Could you check a few things on this model? Use its own coordinates, in mm. A direction names the side the tool comes from. Give positions to 0.01 mm unless a question says otherwise; leave off trailing zeros. Order: outer loops, then holes, each group sorted by start corner. A loop starts at its lowest first (then second) coordinate and runs counter-clockwise, first axis right, second up. Notation, with made-up numbers: (46, 45.25) -> (75, 45.25) arc R21 cw to (75, 62.25) -> close; hole circle Ø5 at (-27.75, -1.5). An arc over 180 degrees is marked (long way). One line per item, written item: value.
```python
from build123d import *

# Parameters (mm, degrees)
F1_DEPTH = 12.7


with BuildPart() as f1:
    # F0 (on Front) → F1 (new body)
    with BuildSketch(Plane.XZ):
        with BuildLine():
            ThreePointArc((13.700902, 62.328232), (6.890739, 63.44321), (0, 63.816324))
            ThreePointArc((0, 63.816324), (-1.449213, 63.799867), (-2.897679, 63.750503))
            ThreePointArc((-2.897679, 63.750503), (-9.764368, 63.06489), (-16.51688, 61.641836))
            ThreePointArc((-16.51688, 61.641836), (-17.912453, 61.250855), (-19.298787, 60.828283))
            ThreePointArc((-19.298787, 60.828283), (-25.75405, 58.388801), (-31.908162, 55.266558))
            ThreePointArc((-31.908162, 55.266558), (-33.154989, 54.527699), (-34.384715, 53.760716))
            ThreePointArc((-34.384715, 53.760716), (-39.988636, 49.733612), (-45.124956, 45.124956))
            ThreePointArc((-45.124956, 45.124956), (-46.138067, 44.08857), (-47.127381, 43.029445))
            ThreePointArc((-47.127381, 43.029445), (-51.498062, 37.68916), (-55.266558, 31.908162))
            ThreePointArc((-55.266558, 31.908162), (-55.976912, 30.644878), (-56.658395, 29.365788))
            ThreePointArc((-56.658395, 29.365788), (-59.497981, 23.076254), (-61.641836, 16.51688))
            ThreePointArc((-61.641836, 16.51688), (-62.001023, 15.112788), (-62.328232, 13.700902))
            ThreePointArc((-62.328232, 13.700902), (-63.44321, 6.890739), (-63.816324, 0))
            ThreePointArc((-63.816324, 0), (-63.799867, -1.449213), (-63.750503, -2.897679))
            ThreePointArc((-63.750503, -2.897679), (-63.06489, -9.764368), (-61.641836, -16.51688))
            ThreePointArc((-61.641836, -16.51688), (-61.250855, -17.912453), (-60.828283, -19.298787))
            ThreePointArc((-60.828283, -19.298787), (-58.388801, -25.75405), (-55.266558, -31.908162))
            ThreePointArc((-55.266558, -31.908162), (-54.527699, -33.154989), (-53.760716, -34.384715))
            ThreePointArc((-53.760716, -34.384715), (-49.733612, -39.988636), (-45.124956, -45.124956))
            ThreePointArc((-45.124956, -45.124956), (-44.08857, -46.138067), (-43.029445, -47.127381))
            ThreePointArc((-43.029445, -47.127381), (-37.68916, -51.498062), (-31.908162, -55.266558))
            ThreePointArc((-31.908162, -55.266558), (-30.644878, -55.976912), (-29.365788, -56.658395))
            ThreePointArc((-29.365788, -56.658395), (-23.076254, -59.497981), (-16.51688, -61.641836))
            ThreePointArc((-16.51688, -61.641836), (-15.112788, -62.001023), (-13.700902, -62.328232))
            ThreePointArc((-13.700902, -62.328232), (-6.890739, -63.44321), (0, -63.816324))
            ThreePointArc((0, -63.816324), (1.449213, -63.799867), (2.897679, -63.750503))
            ThreePointArc((2.897679, -63.750503), (9.764368, -63.06489), (16.51688, -61.641836))
            ThreePointArc((16.51688, -61.641836), (17.912453, -61.250855), (19.298787, -60.828283))
            ThreePointArc((19.298787, -60.828283), (25.75405, -58.388801), (31.908162, -55.266558))
            ThreePointArc((31.908162, -55.266558), (33.154989, -54.527699), (34.384715, -53.760716))
            ThreePointArc((34.384715, -53.760716), (39.988636, -49.733612), (45.124956, -45.124956))
            ThreePointArc((45.124956, -45.124956), (46.138067, -44.08857), (47.127381, -43.029445))
            ThreePointArc((47.127381, -43.029445), (51.498062, -37.68916), (55.266558, -31.908162))
            ThreePointArc((55.266558, -31.908162), (55.976912, -30.644878), (56.658395, -29.365788))
            ThreePointArc((56.658395, -29.365788), (59.497981, -23.076254), (61.641836, -16.51688))
            ThreePointArc((61.641836, -16.51688), (62.001023, -15.112788), (62.328232, -13.700902))
            ThreePointArc((62.328232, -13.700902), (63.44321, -6.890739), (63.816324, 0))
            ThreePointArc((63.816324, 0), (63.799867, 1.449213), (63.750503, 2.897679))
            ThreePointArc((63.750503, 2.897679), (63.06489, 9.764368), (61.641836, 16.51688))
            ThreePointArc((61.641836, 16.51688), (61.250855, 17.912453), (60.828283, 19.298787))
            ThreePointArc((60.828283, 19.298787), (58.388801, 25.75405), (55.266558, 31.908162))
            ThreePointArc((55.266558, 31.908162), (54.527699, 33.154989), (53.760716, 34.384715))
            ThreePointArc((53.760716, 34.384715), (49.733612, 39.988636), (45.124956, 45.124956))
            ThreePointArc((45.124956, 45.124956), (44.08857, 46.138067), (43.029445, 47.127381))
            ThreePointArc((43.029445, 47.127381), (37.68916, 51.498062), (31.908162, 55.266558))
            ThreePointArc((31.908162, 55.266558), (30.644878, 55.976912), (29.365788, 56.658395))
            ThreePointArc((29.365788, 56.658395), (23.076254, 59.497981), (16.51688, 61.641836))
            ThreePointArc((16.51688, 61.641836), (15.112788, 62.001023), (13.700902, 62.328232))
        make_face()
        with BuildLine():
            ThreePointArc((-45.124956, 45.124956), (-39.988636, 49.733612), (-34.384715, 53.760716))
            Line((-34.384715, 53.760716), (-53.916988, 53.916988))
            Line((-53.916988, 53.916988), (-45.124956, 45.124956))
        make_face()
        with BuildLine():
            ThreePointArc((-31.908162, 55.266558), (-25.75405, 58.388801), (-19.298787, 60.828283))
            Line((-19.298787, 60.828283), (-38.125068, 66.034555))
            Line((-38.125068, 66.034555), (-31.908162, 55.266558))
        make_face()
        with BuildLine():
            ThreePointArc((-16.51688, 61.641836), (-9.764368, 63.06489), (-2.897679, 63.750503))
            Line((-2.897679, 63.750503), (-19.734987, 73.651976))
            Line((-19.734987, 73.651976), (-16.51688, 61.641836))
        make_face()
        with BuildLine():
            Line((0, 76.250136), (0, 63.816324))
            ThreePointArc((0, 63.816324), (6.890739, 63.44321), (13.700902, 62.328232))
            Line((13.700902, 62.328232), (0, 76.250136))
        make_face()
        with BuildLine():
            Line((19.734987, 73.651976), (16.51688, 61.641836))
            ThreePointArc((16.51688, 61.641836), (23.076254, 59.497981), (29.365788, 56.658395))
            Line((29.365788, 56.658395), (19.734987, 73.651976))
        make_face()
        with BuildLine():
            Line((38.125068, 66.034555), (31.908162, 55.266558))
            ThreePointArc((31.908162, 55.266558), (37.68916, 51.498062), (43.029445, 47.127381))
            Line((43.029445, 47.127381), (38.125068, 66.034555))
        make_face()
        with BuildLine():
            Line((53.916988, 53.916988), (45.124956, 45.124956))
            ThreePointArc((45.124956, 45.124956), (49.733612, 39.988636), (53.760716, 34.384715))
            Line((53.760716, 34.384715), (53.916988, 53.916988))
        make_face()
        with BuildLine():
            Line((66.034555, 38.125068), (55.266558, 31.908162))
            ThreePointArc((55.266558, 31.908162), (58.388801, 25.75405), (60.828283, 19.298787))
            Line((60.828283, 19.298787), (66.034555, 38.125068))
        make_face()
        with BuildLine():
            Line((73.651976, 19.734987), (61.641836, 16.51688))
            ThreePointArc((61.641836, 16.51688), (63.06489, 9.764368), (63.750503, 2.897679))
            Line((63.750503, 2.897679), (73.651976, 19.734987))
        make_face()
        with BuildLine():
            Line((76.250136, 0), (63.816324, 0))
            ThreePointArc((63.816324, 0), (63.44321, -6.890739), (62.328232, -13.700902))
            Line((62.328232, -13.700902), (76.250136, 0))
        make_face()
        with BuildLine():
            Line((73.651976, -19.734987), (61.641836, -16.51688))
            ThreePointArc((61.641836, -16.51688), (59.497981, -23.076254), (56.658395, -29.365788))
            Line((56.658395, -29.365788), (73.651976, -19.734987))
        make_face()
        with BuildLine():
            Line((66.034555, -38.125068), (55.266558, -31.908162))
            ThreePointArc((55.266558, -31.908162), (51.498062, -37.68916), (47.127381, -43.029445))
            Line((47.127381, -43.029445), (66.034555, -38.125068))
        make_face()
        with BuildLine():
            Line((53.916988, -53.916988), (45.124956, -45.124956))
            ThreePointArc((45.124956, -45.124956), (39.988636, -49.733612), (34.384715, -53.760716))
            Line((34.384715, -53.760716), (53.916988, -53.916988))
        make_face()
        with BuildLine():
            Line((38.125068, -66.034555), (31.908162, -55.266558))
            ThreePointArc((31.908162, -55.266558), (25.75405, -58.388801), (19.298787, -60.828283))
            Line((19.298787, -60.828283), (38.125068, -66.034555))
        make_face()
        with BuildLine():
            Line((19.734987, -73.651976), (16.51688, -61.641836))
            ThreePointArc((16.51688, -61.641836), (9.764368, -63.06489), (2.897679, -63.750503))
            Line((2.897679, -63.750503), (19.734987, -73.651976))
        make_face()
        with BuildLine():
            ThreePointArc((0, -63.816324), (-6.890739, -63.44321), (-13.700902, -62.328232))
            Line((-13.700902, -62.328232), (0, -76.250136))
            Line((0, -76.250136), (0, -63.816324))
        make_face()
        with BuildLine():
            ThreePointArc((-16.51688, -61.641836), (-23.076254, -59.497981), (-29.365788, -56.658395))
            Line((-29.365788, -56.658395), (-19.734987, -73.651976))
            Line((-19.734987, -73.651976), (-16.51688, -61.641836))
        make_face()
        with BuildLine():
            ThreePointArc((-31.908162, -55.266558), (-37.68916, -51.498062), (-43.029445, -47.127381))
            Line((-43.029445, -47.127381), (-38.125068, -66.034555))
            Line((-38.125068, -66.034555), (-31.908162, -55.266558))
        make_face()
        with BuildLine():
            ThreePointArc((-55.266558, -31.908162), (-58.388801, -25.75405), (-60.828283, -19.298787))
            Line((-60.828283, -19.298787), (-66.034555, -38.125068))
            Line((-66.034555, -38.125068), (-55.266558, -31.908162))
        make_face()
        with BuildLine():
            ThreePointArc((-61.641836, -16.51688), (-63.06489, -9.764368), (-63.750503, -2.897679))
            Line((-63.750503, -2.897679), (-73.651976, -19.734987))
            Line((-73.651976, -19.734987), (-61.641836, -16.51688))
        make_face()
        with BuildLine():
            ThreePointArc((-63.816324, 0), (-63.44321, 6.890739), (-62.328232, 13.700902))
            Line((-62.328232, 13.700902), (-76.250136, 0))
            Line((-76.250136, 0), (-63.816324, 0))
        make_face()
        with BuildLine():
            ThreePointArc((-61.641836, 16.51688), (-59.497981, 23.076254), (-56.658395, 29.365788))
            Line((-56.658395, 29.365788), (-73.651976, 19.734987))
            Line((-73.651976, 19.734987), (-61.641836, 16.51688))
        make_face()
        with BuildLine():
            ThreePointArc((-55.266558, 31.908162), (-51.498062, 37.68916), (-47.127381, 43.029445))
            Line((-47.127381, 43.029445), (-66.034555, 38.125068))
            Line((-66.034555, 38.125068), (-55.266558, 31.908162))
        make_face()
        with BuildLine():
            ThreePointArc((-45.124956, -45.124956), (-49.733612, -39.988636), (-53.760716, -34.384715))
            Line((-53.760716, -34.384715), (-53.916988, -53.916988))
            Line((-53.916988, -53.916988), (-45.124956, -45.124956))
        make_face()
    extrude(amount=F1_DEPTH)


solid = f1.part
```
1) Suppose I cut it at C-C, the plane z = 41. Write out the boundary of the cut face in (x, y).
Answer below:
outline: (-54.95, -12.7) -> (53.81, -12.7) -> (53.81, 0) -> (-54.95, 0) -> close
2) Suppose I cut it at A-A, the plane z = -50.5. Write out the boundary of the cut face in (x, y).
Answer below:
outline: (-53.89, -12.7) -> (-50.5, -12.7) -> (-50.5, 0) -> (-53.89, 0) -> close; (-42.15, -12.7) -> (50.5, -12.7) -> (50.5, 0) -> (-42.15, 0) -> close
3) For P1, Ø3, axis at y = -7, z = 58, coming from the -X side; P2, Ø6, axis at y = -9, z = 68.5, coming from the -X side; P3, Ø6, axis at y = -2, z = -7.5, coming from the -X side, each with a flat end and sliding along its axis, tell me the tip position at first contact or that it passes through.
Answer below:
P1: stops at x = -34.35
P2: stops at x = -38.13
P3: stops at x = -68.22
4) We'd pull the mould along X, two halves only. Please class faces 4 (the flat face through (50, -6, -50)), 5 (the flat face through (-60.726, -6.261, -35.06)), 6 (the flat face through (-1, 0, 1)): +X half, -X half, draft (parallel to the pull), parting line (faces both ways), or undercut.
Answer below:
face 4: +X half
face 5: undercut
face 6: draft
5) For faces 1 (the flat face through (60.726, -6.261, 35.06)), 2 (the flat face through (-35.06, -6.261, -60.726)), 3 (the flat face through (-35.06, -6.261, 60.726)), which set-ups out of +Z, -Z, +X, -X, +Y, -Y let a thin tool reach every point of the face, with its end or its side?
Answer below:
face 1: +Z, +Y, -Y
face 2: -Z, +Y, -Y
face 3: -X, +Y, -Y
6) Suppose I cut it at B-B, the plane z = -21.5. Write out the boundary of the cut face in (x, y), then the cut area to 3 significant figures.
Answer below:
outline: (-61.44, -12.7) -> (70.54, -12.7) -> (70.54, 0) -> (-61.44, 0) -> close
area: 1,680 mm2
7) If I drill on line 1 along Z through (x, y) = (36, -2.25); line 2 along Z through (x, y) = (-47.5, -0.75); line 3 along X through (y, z) = (-6.75, 32), over which ranges is the centre line in solid material (lowest first)?
Answer below:
line 1: z = -65.45 to -62.35, -53.77 to 62.35
line 2: z = -47.5 to 42.93, 47.5 to 53.87
line 3: x = -55.43 to 55.21, 55.43 to 64.34
